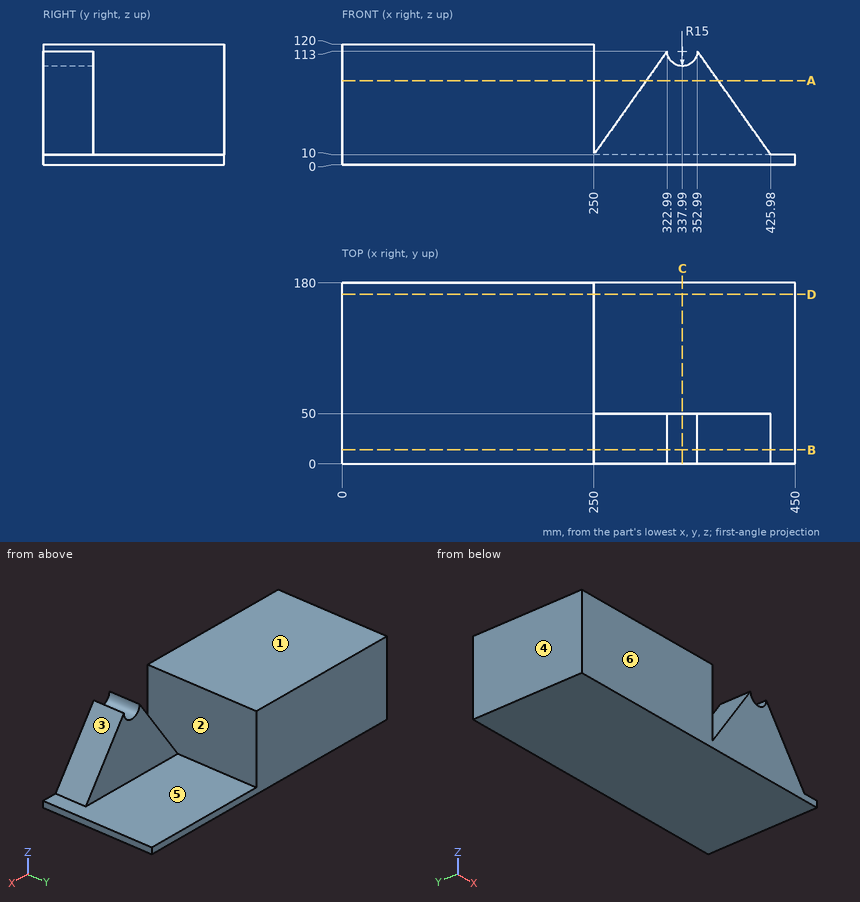
For this review, use the dimensioned drawing (mm, ordinates from the lowest corner) and the shaded views. A direction names the side the tool comes from. Give positions to 0.01 mm unless a question says otherwise; leave off trailing zeros. Order: outer loops, then holes, each group sorted by start corner. A loop starts at its lowest first (then second) coordinate and runs counter-clockwise, first axis right, second up. Notation, with made-up numbers: (8, -10.5) - (62, -10.5) arc R17 ccw to (62, 17.5) - close; hole circle Ø1 at (-31, -34). An arc over 180 degrees is marked (long way). Write item = value, one per line. Start each with the question number.
Q1. We need section D-D on y = 168.5. State the section outline as (x, z) points, plus the area to 3 significant figures.
Q2. We need section C-C on x = 337.99. State the section outline as (y, z) points, plus the area to 3 significant figures.
Q3. We need section A-A on z = 83.5. State the section outline as (x, y) points.
Q4. Mouldability with a two-part tool opening along X and no side actions: class the marked faces 1, 2, 3 and 4 as released by +X, released by -X, zero draft, split by the parting line, or undercut.
Q5. We need section B-B on y = 14. State the section outline as (x, z) points, plus the area to 3 significant figures.
Q6. To check wall thickness, follow L1, parallel to Z at x = 365.5, y = 167; L2, parallel to X at y = 130.5, z = 57.5; L3, parallel to X at y = 32, z = 43.5. State the ranges of each line that lie inside material, in increasing order. Write a range as from..to.
Q7. Clearance check with a flat-ended pin moving along its axis: pin 1 Ø5 at (y, z) = (159, 26) entering from +X. State where the tip first meets the part, or that it passes through.
Q8. Tool access review of the marked faces 5 and 6: name each direction out of +Z, -Z, +X, -X, +Y, -Y from which nothing blocks a thin tool from reaching the whole face with its end or side.
Working result:
q1.outline = (0, 0) - (450, 0) - (450, 10) - (250, 10) - (250, 120) - (0, 120) - close
q1.area = 32,000 mm²
q2.outline = (0, 0) - (180, 0) - (180, 10) - (50, 10) - (50, 98) - (0, 98) - close
q2.area = 6,200 mm²
q3.outline = (0, 0) - (250, 0) - (250, 180) - (0, 180) - close; (302.09, 0) - (373.89, 0) - (373.89, 50) - (302.09, 50) - close
q4.face_1 = zero draft
q4.face_2 = undercut
q4.face_3 = released by +X
q4.face_4 = released by -X
q5.outline = (0, 0) - (450, 0) - (450, 10) - (425.98, 10) - (352.99, 113) arc R15 cw to (322.99, 113) - (250, 10) - (250, 120) - (0, 120) - close
q5.area = 42,300 mm²
q6.L1 = 0..10
q6.L2 = 0..250
q6.L3 = 0..250, 273.74..402.24
q7.pin_1 = 250
q8.face_5 = +Z, +X, +Y
q8.face_6 = +Z, -Z, +X, -X, -Y
